from build123d import *

# Parameters (mm, degrees)
MAIN_EXTRUSION_DEPTH             = 14
TAPERED_BOTTOM_DEPTH             = 2
TAPERED_BOTTOM_DRAFT             = -45
SKETCH4_R                        = 2.795
SKETCH4_W                        = 8
SKETCH4_H                        = 3.045
PCB_SUPPORT_DEPTH                = 13.75
SKETCH5_R                        = 2.045
GUIDE_PIN_CUTOUT_DEPTH           = 2
GUIDE_PIN_CUTOUT_DRAFT           = 7.5
GUIDE_PIN_CUTOUT_PROFILE_2_DEPTH = 2
GUIDE_PIN_CUTOUT_PROFILE_2_DRAFT = 7.5
SKETCH12_W                       = 4.994797294
SKETCH12_H                       = 14
CUT_EXTRUDE6_DEPTH               = 13.75
SKETCH11_W                       = 7
SKETCH11_H                       = 7
BOSS_EXTRUDE1_DEPTH              = 2
CUT_EXTRUDE2_REACH               = 48.243
SKETCH8_R                        = 6.5
CUT_EXTRUDE4_DEPTH               = 0.5
CUT_EXTRUDE5_REACH               = 48.243
CHAMFER1_SIZE                    = 0.5


with BuildPart() as part:
    # Sketch2 → main-extrusion (new body)
    with BuildSketch(Plane(origin=(0, 0, 0), x_dir=(1, 0, 0), z_dir=(0, 1, 0))):
        with BuildLine():
            Line((-2.25, 19.36), (-2.25, 2.23))
            ThreePointArc((-2.25, 2.23), (-0.93783838, -0.93783838), (2.23, -2.25))
            Line((2.23, -2.25), (29.52, -2.25))
            ThreePointArc((29.52, -2.25), (32.68783838, -0.93783838), (34, 2.23))
            Line((34, 2.23), (34, 19.36))
            ThreePointArc((34, 19.36), (32.68783838, 22.52783838), (29.52, 23.84))
            Line((29.52, 23.84), (2.23, 23.84))
            ThreePointArc((2.23, 23.84), (-0.93783838, 22.52783838), (-2.25, 19.36))
        make_face()
        with BuildLine():
            Line((-0.25, 19.36), (-0.25, 2.23))
            ThreePointArc((-0.25, 2.23), (0.476375183, 0.476375183), (2.23, -0.25))
            Line((2.23, -0.25), (29.52, -0.25))
            ThreePointArc((29.52, -0.25), (31.273624817, 0.476375183), (32, 2.23))
            Line((32, 2.23), (32, 19.36))
            ThreePointArc((32, 19.36), (31.273624817, 21.113624817), (29.52, 21.84))
            Line((29.52, 21.84), (2.23, 21.84))
            ThreePointArc((2.23, 21.84), (0.476375183, 21.113624817), (-0.25, 19.36))
        make_face(mode=Mode.SUBTRACT)
    extrude(amount=MAIN_EXTRUSION_DEPTH)


with BuildPart() as tapered_bottom_tool:
    # Sketch3 → tapered-bottom (with draft: the straight prism first)
    with BuildSketch(Plane.XZ.offset(-14)):
        with BuildLine():
            ThreePointArc((-2.25, -19.36), (-0.93783838, -22.52783838), (2.23, -23.84))
            Line((2.23, -23.84), (29.52, -23.84))
            ThreePointArc((29.52, -23.84), (32.68783838, -22.52783838), (34, -19.36))
            Line((34, -19.36), (34, -2.23))
            ThreePointArc((34, -2.23), (32.68783838, 0.93783838), (29.52, 2.25))
            Line((29.52, 2.25), (2.23, 2.25))
            ThreePointArc((2.23, 2.25), (-0.93783838, 0.93783838), (-2.25, -2.23))
            Line((-2.25, -2.23), (-2.25, -19.36))
        make_face()
    extrude(amount=-TAPERED_BOTTOM_DEPTH)
    # tapered-bottom: the draft: its side faces are tilted about the plane it starts from
    tapered_bottom_sides = [tapered_bottom_tool.faces().sort_by_distance(p)[0] for p in [
        (-0.93783838, 15, -22.52783838),
        (15.875, 15, -23.84),
        (32.68783838, 15, -22.52783838),
        (34, 15, -10.795),
        (32.68783838, 15, 0.93783838),
        (15.875, 15, 2.25),
        (-0.93783838, 15, 0.93783838),
        (-2.25, 15, -10.795),
    ]]
    draft(tapered_bottom_sides, Plane.XZ.offset(-14), TAPERED_BOTTOM_DRAFT)


with BuildPart() as part_1:
    add(part.part)

    # tapered-bottom: add tapered_bottom_tool
    add(tapered_bottom_tool.part)

    # Sketch4 → PCB-support (add)
    with BuildSketch(Plane(origin=(0, 14, 0), x_dir=(1, 0, 0), z_dir=(0, 1, 0))):
        with Locations((27.94, 19.05)):
            Circle(SKETCH4_R)
        with Locations((27.94, 2.54)):
            Circle(SKETCH4_R)
        with Locations((13, 20.3175)):
            Rectangle(SKETCH4_W, SKETCH4_H)
        with Locations((13, 1.2725)):
            Rectangle(SKETCH4_W, SKETCH4_H)
    extrude(amount=-PCB_SUPPORT_DEPTH)


with BuildPart() as guide_pin_cutout_tool:
    # Sketch5 → guide-pin-cutout (with draft: the straight prism first)
    with BuildSketch(Plane(origin=(0, 0, 0), x_dir=(1, 0, 0), z_dir=(0, 1, 0))):
        with Locations((27.94, 19.05)):
            Circle(SKETCH5_R)
    extrude(amount=GUIDE_PIN_CUTOUT_DEPTH)
    # guide-pin-cutout: the draft: its side faces are tilted about the plane it starts from
    guide_pin_cutout_sides = [guide_pin_cutout_tool.faces().sort_by_distance(p)[0] for p in [
        (25.895, 1, -19.05),
    ]]
    draft(guide_pin_cutout_sides, Plane(origin=(0, 0, 0), x_dir=(1, 0, 0), z_dir=(0, 1, 0)), GUIDE_PIN_CUTOUT_DRAFT)


with BuildPart() as part_2:
    add(part_1.part)

    # guide-pin-cutout: cut by guide_pin_cutout_tool
    add(guide_pin_cutout_tool.part, mode=Mode.SUBTRACT)


with BuildPart() as guide_pin_cutout_profile_2_tool:
    # Sketch5 → guide-pin-cutout profile 2 (with draft: the straight prism first)
    with BuildSketch(Plane(origin=(0, 0, 0), x_dir=(1, 0, 0), z_dir=(0, 1, 0))):
        with Locations((27.94, 2.54)):
            Circle(SKETCH5_R)
    extrude(amount=GUIDE_PIN_CUTOUT_PROFILE_2_DEPTH)
    # guide-pin-cutout profile 2: the draft: its side faces are tilted about the plane it starts from
    guide_pin_cutout_profile_2_sides = [guide_pin_cutout_profile_2_tool.faces().sort_by_distance(p)[0] for p in [
        (25.895, 1, -2.54),
    ]]
    draft(guide_pin_cutout_profile_2_sides, Plane(origin=(0, 0, 0), x_dir=(1, 0, 0), z_dir=(0, 1, 0)), GUIDE_PIN_CUTOUT_PROFILE_2_DRAFT)


with BuildPart() as part_3:
    add(part_2.part)

    # guide-pin-cutout profile 2: cut by guide_pin_cutout_profile_2_tool
    add(guide_pin_cutout_profile_2_tool.part, mode=Mode.SUBTRACT)

    # Sketch12 → Cut-Extrude6 (cut)
    with BuildSketch(Plane.XZ.offset(-14)):
        with Locations((27.94, -10.795)):
            Rectangle(SKETCH12_W, SKETCH12_H)
    extrude(amount=CUT_EXTRUDE6_DEPTH, mode=Mode.SUBTRACT)

    # Sketch11 → Boss-Extrude1 (add)
    with BuildSketch(Plane.XZ.offset(-14)):
        with Locations((28.5, -10.795)):
            Rectangle(SKETCH11_W, SKETCH11_H)
    extrude(amount=BOSS_EXTRUDE1_DEPTH)

    # top-hook: sweep along a path in path
    with BuildLine(Plane.XZ) as top_hook_path:
        Line((2.23, 0.25), (29.52, 0.25))
        ThreePointArc((29.52, 0.25), (31.273624817, -0.476375183), (32, -2.23))
        Line((32, -2.23), (32, -19.36))
        ThreePointArc((32, -19.36), (31.273624817, -21.113624817), (29.52, -21.84))
        Line((29.52, -21.84), (2.23, -21.84))
        ThreePointArc((2.23, -21.84), (0.476375183, -21.113624817), (-0.25, -19.36))
        Line((-0.25, -19.36), (-0.25, -2.23))
        ThreePointArc((-0.25, -2.23), (0.476375183, -0.476375183), (2.23, 0.25))
    # hook → top-hook (sweep)
    with BuildSketch(Plane(origin=(29.52, 0, 0), x_dir=(0, 0, -1), z_dir=(1, 0, 0))):
        with BuildLine():
            Line((22.84, -2.9), (22.84, -1.3))
            ThreePointArc((22.84, -1.3), (23.19, -0.75), (22.84, -0.2))
            Line((22.84, -0.2), (22.84, 0))
            Line((22.84, 0), (23.84, 0))
            Line((23.84, 0), (23.84, -2.9))
            Line((23.84, -2.9), (22.84, -2.9))
        make_face()
    sweep(path=top_hook_path.line)

    # Sketch8 → Cut-Extrude2 (cut, up to next)
    with BuildSketch(Plane.ZY.offset(2.25), mode=Mode.PRIVATE) as cut_extrude2_sk1:
        with Locations((-10.795, 7)):
            Circle(SKETCH8_R)
    cut_extrude2_tool1 = extrude(cut_extrude2_sk1.sketch, amount=-CUT_EXTRUDE2_REACH, mode=Mode.PRIVATE) & part_3.part
    add(cut_extrude2_tool1.solids().sort_by_distance((-2.25, 7, -10.795))[0], mode=Mode.SUBTRACT)

    # Sketch9 → Cut-Extrude4 (cut)
    with BuildSketch(Plane.ZY.offset(2.25)):
        with BuildLine():
            Line((-18.295, 7), (-18.295, 12))
            ThreePointArc((-18.295, 12), (-17.709213562, 13.414213562), (-16.295, 14))
            Line((-16.295, 14), (-5.295, 14))
            ThreePointArc((-5.295, 14), (-3.880786438, 13.414213562), (-3.295, 12))
            Line((-3.295, 12), (-3.295, 7))
            ThreePointArc((-3.295, 7), (-10.795, -0.5), (-18.295, 7))
        make_face()
    extrude(amount=-CUT_EXTRUDE4_DEPTH, mode=Mode.SUBTRACT)

    # Sketch10 → Cut-Extrude5 (cut, up to next)
    with BuildSketch(Plane(origin=(34, 0, 0), x_dir=(0, 0, -1), z_dir=(1, 0, 0)), mode=Mode.PRIVATE) as cut_extrude5_sk1:
        Polygon((5.295, 1), (16.295, 1), (16.295, 10), (14.295, 12), (7.295, 12), (5.295, 10), align=None)
    cut_extrude5_tool1 = extrude(cut_extrude5_sk1.sketch, amount=-CUT_EXTRUDE5_REACH, mode=Mode.PRIVATE) & part_3.part
    add(cut_extrude5_tool1.solids().sort_by_distance((34, 6.334758, -10.795))[0], mode=Mode.SUBTRACT)

    # Chamfer1
    chamfer1_edges = [part_3.edges().sort_by_distance(p)[0] for p in [
        (15.875, -2.9, -22.84),
        (-0.230731599, -2.9, -21.820731599),
        (-1.25, -2.9, -10.795),
        (-0.230731599, -2.9, 0.230731599),
        (15.875, -2.9, 1.25),
        (31.980731599, -2.9, 0.230731599),
        (33, -2.9, -10.795),
        (31.980731599, -2.9, -21.820731599),
    ]]
    chamfer(chamfer1_edges, length=CHAMFER1_SIZE)


solid = part_3.part
Design review of the part built by this model. Coordinates are the model's own, in mm. A direction names the side the tool comes from. Coordinates: 2 decimals unless noted, no trailing zeros. Write each loop counter-clockwise with the first axis right and the second up, starting at its lowest first coordinate (ties: lowest second). Pieces come first, ordered by that corner, then holes. Notation, with made-up numbers: (46, 55) -> (76, 55) arc R19 cw to (76, 71) -> close; hole circle Ø2 at (4.25, 42.25). An arc over 180 degrees is marked (long way). Write each question's results on one line, items separated by ' | '. Start each with the question number.
(1) The part is to be moulded in two halves that separate along Z. For faces 1 (the face through (33, 6, -5.295)), 2 (the face through (-0.109, 15.208, -21.648)), say which applies: pulls with the +Z half, pulls with the -Z half, needs draft (parallel to the pull), parting line crosses it, or undercut.
(2) Take a section at A-A on x = 18. Write out the cut boundary in (y, z), and give its area (3 significant figures).
(3) For line 1 along Z through (x, y) = (15.5, 9.75) (3 decimals); line 2 along X through (y, z) = (4.5, -21.25); line 3 along X through (y, z) = (12.5, -15.5), list the stretches that pass through material, from the lowest coordinate up. Write a range as from..to.
(4) Tool access review of faces 3 (the face through (-1.01, 8.952, -4.595)), 4 (the face through (28, 7, -3.795)): name each direction out of +Z, -Z, +X, -X, +Y, -Y from which nothing blocks a thin tool from reaching the whole face with its end or side.
(5) Clearance check with flat-ended pins moving along their axes: P1, Ø5, axis at x = 18.5, z = -9, coming from the -Y side; P2, Ø7, axis at y = 5.5, z = -8.5, coming from the +X side; P3, Ø2.5, axis at x = 15, z = -20, coming from the -Y side; P4, Ø1.6, axis at x = 33.5, z = -9, coming from the +Y side. State where each tip first meets the part, or that it passes through.
(6) Take a section at B-B on z = -13.5. Give the number of separate pieces and of enclosed holes in the cut face, and give its area (3 significant figures).
Results found:
1) face 1: undercut | face 2: pulls with the -Z half
2) outline: (-2.9, -23.84) -> (14, -23.84) -> (16, -21.84) -> (16, 0.25) -> (14, 2.25) -> (-2.9, 2.25) -> (-2.9, 1.75) -> (-2.4, 1.25) -> (-1.3, 1.25) arc R0.61 cw to (-0.2, 1.25) -> (0, 1.25) -> (0, 0.25) -> (14, 0.25) -> (14, -21.84) -> (0, -21.84) -> (0, -22.84) -> (-0.2, -22.84) arc R0.61 cw to (-1.3, -22.84) -> (-2.4, -22.84) -> (-2.9, -23.34) -> close | area: 109 mm2
3) line 1: z = -23.84..-18.795, -2.795..2.25 | line 2: x = -1.83..0.62, 9..17, 26.22..29.66, 31.13..33.58 | line 3: x = -1.75..-0.25, 32..34
4) face 3: -X | face 4: -Y
5) P1: stops at y = 14 | P2: stops at x = 34 | P3: stops at y = 0.25 | P4: stops at y = 15.3
6) separate pieces: 3 | enclosed holes: 0 | area: 96.8 mm2
